```python
from build123d import *

# Parameters (mm, degrees)
ESQUISSE1_W             = 49
ESQUISSE1_H             = 49
ESQUISSE1_W_2           = 43
ESQUISSE1_H_2           = 43
ESQUISSE1_R             = 3.5
BOSS_EXTRU_1_DEPTH      = 4
ESQUISSE2_W             = 49
ESQUISSE2_H             = 49
ESQUISSE2_W_2           = 43
ESQUISSE2_H_2           = 43
BOSS_EXTRU_2_DEPTH      = 38
ESQUISSE3_W             = 14
ESQUISSE3_H             = 42
ENL_V_MAT_EXTRU_1_DEPTH = 3
ESQUISSE4_W             = 14
ESQUISSE4_H             = 4
BOSS_EXTRU_3_DEPTH      = 3


with BuildPart() as part:
    # Esquisse1 → Boss.-Extru.1 (new body)
    with BuildSketch(Plane(origin=(0, 0, 0), x_dir=(1, 0, 0), z_dir=(0, 1, 0))):
        with Locations((21.5, 21.5)):
            Rectangle(ESQUISSE1_W, ESQUISSE1_H)
        with Locations((21.5, 21.5)):
            Rectangle(ESQUISSE1_W_2, ESQUISSE1_H_2, mode=Mode.SUBTRACT)
        with Locations((21.5, 21.5)):
            Rectangle(ESQUISSE1_W_2, ESQUISSE1_H_2)
        with Locations(Location((35.928932188, 7.071067812, 0), (0, 0, 270))):
            Circle(ESQUISSE1_R, mode=Mode.SUBTRACT)
        with Locations(Location((7.071067812, 35.928932188, 0), (0, 0, 270))):
            Circle(ESQUISSE1_R, mode=Mode.SUBTRACT)
    extrude(amount=BOSS_EXTRU_1_DEPTH)

    # Esquisse2 → Boss.-Extru.2 (add)
    with BuildSketch(Plane(origin=(0, 4, 0), x_dir=(1, 0, 0), z_dir=(0, 1, 0))):
        with Locations((21.5, 21.5)):
            Rectangle(ESQUISSE2_W, ESQUISSE2_H)
        with Locations((21.5, 21.5)):
            Rectangle(ESQUISSE2_W_2, ESQUISSE2_H_2, mode=Mode.SUBTRACT)
    extrude(amount=BOSS_EXTRU_2_DEPTH)

    # Esquisse3 → Enlèv. mat.-Extru.1 (cut)
    with BuildSketch(Plane.XY.offset(3)):
        with Locations((21.5, 21)):
            Rectangle(ESQUISSE3_W, ESQUISSE3_H)
    extrude(amount=-ENL_V_MAT_EXTRU_1_DEPTH, mode=Mode.SUBTRACT)

    # Esquisse4 → Boss.-Extru.3 (add)
    with BuildSketch(Plane.XY):
        with Locations((21.5, 2)):
            Rectangle(ESQUISSE4_W, ESQUISSE4_H)
    extrude(amount=BOSS_EXTRU_3_DEPTH)


solid = part.part
```
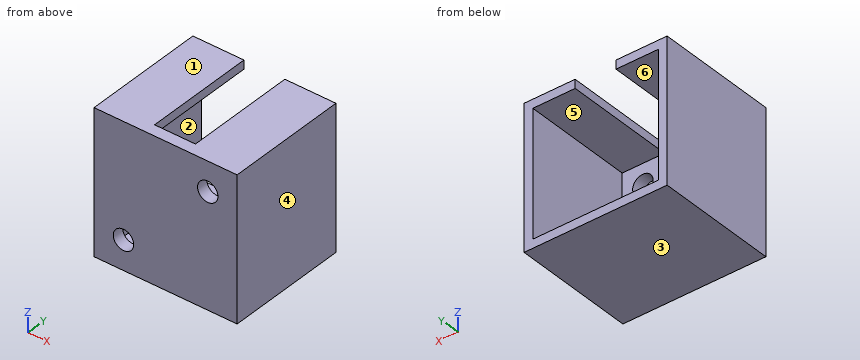
The listing builds one solid part. Answer for the finished solid, in the listing's coordinates (mm). Face numbers are marked on the shaded views. A direction names the side the tool comes from. Give positions to 0.01 mm unless a question says otherwise; leave off trailing zeros. Order: outer loops, then holes, each group sorted by start corner. A loop starts at its lowest first (then second) coordinate and runs counter-clockwise, first axis right, second up. Notation, with made-up numbers: (32.25, 62.5) -> (72.25, 62.5) arc R26 cw to (72.25, 100.5) -> close; hole circle Ø5 at (76, 0). An arc over 180 degrees is marked (long way). Answer as a JSON object with one key per item and string values. Group by question number.
Item 1: The part is cut by section A-A on y = 7. Write down the section's boundary in (x, z).
Item 2: The part is cut by section C-C on z = -30. Write down the section's boundary in (x, y), and give its area (3 significant figures).
Item 3: A tool of negligible diameter and unlimited length cuts with its end or side. For the marked faces 1 and 2, from which of +Z, -Z, +X, -X, +Y, -Y can it reach the whole face along a straight path? Write none if from no direction.
Item 4: The part is cut by section D-D on z = -9.5. Write down the section's boundary in (x, y).
Item 5: Consider L1, parallel to Z at x = 35.5, y = 17.5; L2, parallel to X at y = 16, z = -28; L3, parallel to Y at x = 36.5, z = -38.5. Determine where each line is inside the solid, lowest interval first. Write a range as from..to.
Item 6: The part is cut by section B-B on x = 31. Write down the section's boundary in (y, z).
Item 7: Determine the mould class of the marked faces 3, 4, 5 and 6 for opening direction X: pulls with the +X half, pulls with the -X half, needs draft (parallel to the pull), parting line crosses it, or undercut.
Item 8: A flat-ended cylindrical pin translates along its axis: pin 1 (21.5 mm diameter, centred on x = 21.5, z = -25.5, fed in from +Y). Find the tip coordinate at first contact, or state that the pin passes through.
Result set:
{
 "1": {"outline": "(-3, -46) -> (46, -46) -> (46, 3) -> (28.5, 3) -> (28.5, 0) -> (43, 0) -> (43, -43) -> (0, -43) -> (0, 0) -> (14.5, 0) -> (14.5, 3) -> (-3, 3) -> close"},
 "2": {"outline": "(-3, 0) -> (46, 0) -> (46, 42) -> (43, 42) -> (43, 4) -> (0, 4) -> (0, 42) -> (-3, 42) -> close", "area": "424 mm²"},
 "3": {"face 1": "+Z, +X, -X, +Y, -Y", "face 2": "+Y"},
 "4": {"outline": "(-3, 0) -> (33.41, 0) -> (33.41, 4) -> (0, 4) -> (0, 42) -> (-3, 42) -> close; (38.45, 0) -> (46, 0) -> (46, 42) -> (43, 42) -> (43, 4) -> (38.45, 4) -> close"},
 "5": {"L1": "-46..-43, 0..3", "L2": "-3..0, 43..46", "L3": "0..4"},
 "6": {"outline": "(0, -46) -> (42, -46) -> (42, -43) -> (4, -43) -> (4, 0) -> (42, 0) -> (42, 3) -> (0, 3) -> close"},
 "7": {"face 3": "needs draft", "face 4": "pulls with the +X half", "face 5": "undercut", "face 6": "undercut"},
 "8": {"pin 1": "y = 4"}
}
